Could you check a few things on this drawing? It's one solid part, dimensions in mm from its lowest x, y, z. A direction names the side the tool comes from. Coordinates: 2 decimals unless noted, no trailing zeros. Order: outer loops, then holes, each group sorted by start corner. A loop starts at its lowest first (then second) coordinate and runs counter-clockwise, first axis right, second up. Notation, with made-up numbers: (89.25, -22) - (110.25, -22) arc R21 ccw to (110.25, -10) - close; hole circle Ø6 at (76, 46). An arc over 180 degrees is marked (long way). Return JSON: item names as keys, results as strings. Group by question number.
1) Which directions (+Z, -Z, +X, -X, +Y, -Y) give clear straight access to the entire face, cutting with the end or side of a thin tool? Please do the marked faces 1 and 2.
2) For pin 1 Ø12 at (x, z) = (20, 18.5) entering from -Y, with a flat end and sliding along its axis, tell me the tip position at first contact or that it passes through.
3) If I drill on line 1 along X through (y, z) = (6.5, 30.5); line 2 along Y through (x, z) = (25.5, 18.5), over which ranges is the centre line in solid material (lowest first)?
4) Imagine slicing it at B-B (z = 49). Write out the boundary of the cut face in (x, y), and give its area (3 significant figures).
5) Imagine slicing it at C-C (x = 10.5). Write out the boundary of the cut face in (y, z).
6) Imagine slicing it at A-A (y = 4.25). Write out the boundary of the cut face in (x, z), and give its area (3 significant figures).
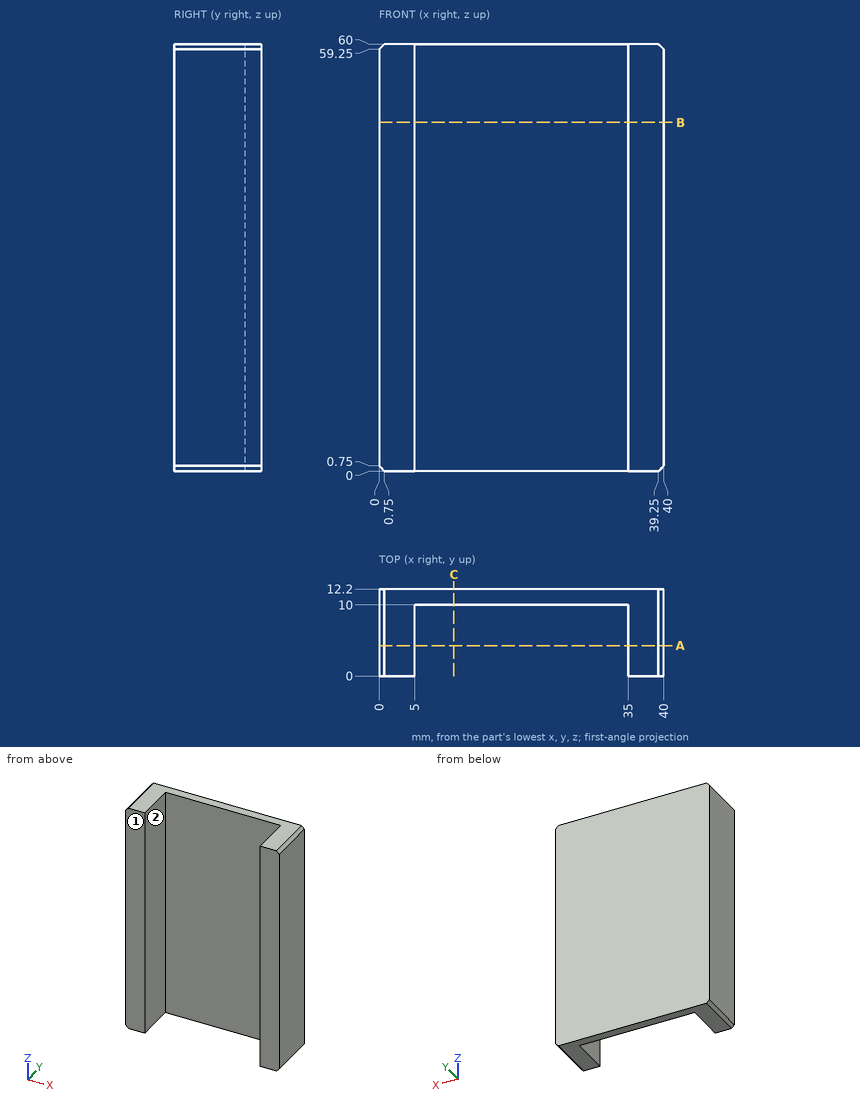
Calculated:
{
 "1": {"face 1": "+Z, -Z, +X, -X, -Y", "face 2": "+Z, -Z, -Y"},
 "2": {"pin 1": "y = 10"},
 "3": {"line 1": "0 to 5, 35 to 40", "line 2": "10 to 12.2"},
 "4": {"outline": "(0, 0) - (5, 0) - (5, 10) - (35, 10) - (35, 0) - (40, 0) - (40, 12.2) - (0, 12.2) - close", "area": "188 mm2"},
 "5": {"outline": "(10, 0) - (12.2, 0) - (12.2, 60) - (10, 60) - close"},
 "6": {"outline": "(0, 0.75) - (0.75, 0) - (5, 0) - (5, 60) - (0.75, 60) - (0, 59.25) - close; (35, 0) - (39.25, 0) - (40, 0.75) - (40, 59.25) - (39.25, 60) - (35, 60) - close", "area": "599 mm2"}
}
